```python
from build123d import *


# Not quite as in the source:
# - a feature names something its author has since deleted; it is built from what else it names


with BuildPart() as f1:
    # F0 (on Front) → F1 (revolve)
    with BuildSketch(Plane.XZ):
        with BuildLine():
            Line((0, 10.7571836561), (0, 0))
            Line((0, 0), (10, 0))
            Line((10, 0), (10, 2))
            Line((10, 2), (9, 2))
            ThreePointArc((9, 2), (9.2928932188, 2.7071067812), (10, 3))
            add(Edge.make_bspline(
                [(10, 3), (4.8616999982, 7.4005079185), (3.2689606671, 13.2153081121), (3.1879616163, 19.0694751767)],
                knots=[0, 0, 0, 0, 0.2884989323, 0.2884989323, 0.2884989323, 0.2884989323], degree=3))
            Line((3.1879616163, 19.0694751767), (0.9205695706, 18.3377522863))
            Line((0.9205695706, 18.3377522863), (0, 10.7571836561))
        make_face()
        with BuildLine():
            Line((0, 51), (0, 44))
            add(Edge.make_bspline(
                [(2.3170218427, 44.2838583015), (1.6508949311, 44.2597847974), (0.8824741052, 44.1653776789), (0, 44)],
                knots=[0.9455867567, 0.9455867567, 0.9455867567, 0.9455867567, 1, 1, 1, 1], degree=3))
            Line((2.3170218427, 44.2838583015), (0, 51))
        make_face()
        with BuildLine():
            Line((1.3255104114, 21.6722985633), (0.9205695706, 18.3377522863))
            Line((0.9205695706, 18.3377522863), (3.1879616163, 19.0694751767))
            add(Edge.make_bspline(
                [(3.1879616163, 19.0694751767), (3.1781161003, 19.7810550677), (3.1906060131, 20.4932165904), (3.2217788711, 21.203490553)],
                knots=[0.2884989323, 0.2884989323, 0.2884989323, 0.2884989323, 0.3235662675, 0.3235662675, 0.3235662675, 0.3235662675], degree=3))
            Line((3.2217788711, 21.203490553), (1.3255104114, 21.6722985633))
        make_face()
        with BuildLine():
            add(Edge.make_bspline(
                [(3.1879616163, 19.0694751767), (3.1781161003, 19.7810550677), (3.1906060131, 20.4932165904), (3.2217788711, 21.203490553)],
                knots=[0.2884989323, 0.2884989323, 0.2884989323, 0.2884989323, 0.3235662675, 0.3235662675, 0.3235662675, 0.3235662675], degree=3))
            Line((3.1879616163, 19.0694751767), (6.9468966685, 20.282542333))
            Line((6.9468966685, 20.282542333), (3.2217788711, 21.203490553))
        make_face()
        with BuildLine():
            Line((1.7987132305, 25.5689583719), (1.3255104114, 21.6722985633))
            Line((1.3255104114, 21.6722985633), (3.2217788711, 21.203490553))
            add(Edge.make_bspline(
                [(3.2217788711, 21.203490553), (3.551315279, 28.7119817542), (7.6075295102, 40.9568023902), (5.393614482, 44.39504487), (2.3170218427, 44.2838583015)],
                knots=[0.3235662675, 0.3235662675, 0.3235662675, 0.3235662675, 0.6942722088, 0.9455867567, 0.9455867567, 0.9455867567, 0.9455867567], degree=3))
            add(Edge.make_bspline(
                [(2.3170218427, 44.2838583015), (1.6508949311, 44.2597847974), (0.8824741052, 44.1653776789), (0, 44)],
                knots=[0.9455867567, 0.9455867567, 0.9455867567, 0.9455867567, 1, 1, 1, 1], degree=3))
            Line((0, 44), (0, 41.3012392819))
            Line((0, 41.3012392819), (3.2213132363, 40.3807349503))
            Line((3.2213132363, 40.3807349503), (3.8907721173, 38.874451071))
            Line((3.8907721173, 38.874451071), (1.7987132305, 25.5689583719))
        make_face()
    revolve(axis=Axis((0, 0, 22), (0, 0, 1)))


solid = f1.part
```
Design review of the part built by this model. Coordinates are the model's own, in mm. A direction names the side the tool comes from. Coordinates: 2 decimals unless noted, no trailing zeros. Order: outer loops, then holes, each group sorted by start corner. A loop starts at its lowest first (then second) coordinate and runs counter-clockwise, first axis right, second up.
1) Wall thickness on line 1 along Z through (x, y) = (-6.25, 2); line 2 along Y through (x, z) = (1, 28); line 3 along X through (y, z) = (-1.25, 26.5): over which ranges is each line inside the solid? List them lowest first.
2) Take a section at A-A, the plane x = -5.5. State how many separate pieces and enclosed holes the cut face has, and give its area (3 significant figures).
3) Clearance check with flat-ended pins moving along their axes: pin 1 (4 mm diameter, centred on x = -0.5, y = 5.5, fed in from +Z); pin 2 (1.5 mm diameter, centred on x = -3, z = 31, fed in from +Y); pin 3 (6 mm diameter, centred on x = 6.5, z = 12.5, fed in from +Y). State where each tip first meets the part, or that it passes through.
4) Take a section at B-B, the plane z = 46.5. Give the boundary of the cut face in (x, y).
5) Mouldability with a two-part tool opening along Y and no side actions: class faces 1 (the conical face through (0.192, 0.061, 41.244)), 2 (the flat face through (0, 0, 0)), 3 (the cylindrical face through (-2.17, -9.76, 1.01)) as +Y half, -Y half, draft (parallel to the pull), parting line (faces both ways), or undercut.
6) For faces 4 (the conical face through (-0.368, 2.806, 32.129)), 5 (the conical face through (-0.15, 1.13, 47.69)), list the 3-axis set-ups (+Z, -Z, +X, -X, +Y, -Y) from which the entire face can be reached by the end or side of a thin tool; tool diameter is ignored.
Returned:
1. line 1: z = 0 to 6.86, 20.16 to 20.38
1. line 2: y = -3.87 to -1.94, 1.94 to 3.87
1. line 3: x = -3.54 to -1.49, 1.49 to 3.54
2. separate pieces: 3
2. enclosed holes: 0
2. area: 139 mm2
3. pin 1: stops at z = 44.24
3. pin 2: stops at y = 3.99
3. pin 3: stops at y = 2.32
4. outline: circle Ø3.1 at (0, 0)
5. face 1: undercut
5. face 2: draft
5. face 3: parting line
6. face 4: none
6. face 5: +Z
